from build123d import *

# Parameters (mm, degrees)
EXTRUDE_1_DEPTH           = 6
FILLET_1_R                = 3
HOLE_WIZARD_2_D           = 4.5
HOLE_WIZARD_2_CBORE_D     = 8
HOLE_WIZARD_2_CBORE_DEPTH = 4.6
CHAMFER_1_SIZE            = 1


with BuildPart() as part:
    # 草图1 → 旋转1 (revolve)
    with BuildSketch(Plane.XY):
        Polygon((-6, 10.5), (-6, 18), (0, 18), (0, 14), (4, 14), (4, 11), (-3, 11), (-3, 10.5), align=None)
    revolve(axis=Axis((-10.541189269, 0, 0), (1, 0, 0)))

    # 草图5 → 凸台-拉伸1 (add)
    with BuildSketch(Plane.ZY.offset(6)):
        with BuildLine():
            ThreePointArc((-2.6e-08, 18), (12.727922052, 12.72792207), (18, 0))
            Line((18, 0), (18, 18))
            Line((18, 18), (-2.6e-08, 18))
        make_face()
        with BuildLine():
            Line((-18, 18), (-18, 3.1e-08))
            ThreePointArc((-18, 3.1e-08), (-12.72792206, 12.727922063), (-2.6e-08, 18))
            Line((-2.6e-08, 18), (-18, 18))
        make_face()
        with BuildLine():
            Line((-18, 3.1e-08), (-18, -18))
            Line((-18, -18), (0, -18))
            ThreePointArc((0, -18), (-12.727922072, -12.727922051), (-18, 3.1e-08))
        make_face()
        with BuildLine():
            ThreePointArc((18, 0), (12.727922061, -12.727922061), (0, -18))
            Line((0, -18), (18, -18))
            Line((18, -18), (18, 0))
        make_face()
    extrude(amount=-EXTRUDE_1_DEPTH)

    # 圆角1
    fillet_1_edges = [part.edges().sort_by_distance(p)[0] for p in [
        (-3, 18, 18),
        (-3, 18, -18),
        (-3, -18, -18),
        (-3, -18, 18),
    ]]
    fillet(fillet_1_edges, radius=FILLET_1_R)

    # 打孔尺寸(%根据)内六角圆柱头螺钉的类型2 (through all)
    with Locations(Plane.ZY.offset(6)):
        with Locations((-13, 13), (13, 13), (13, -13), (-13, -13)):
            CounterBoreHole(HOLE_WIZARD_2_D / 2, HOLE_WIZARD_2_CBORE_D / 2, HOLE_WIZARD_2_CBORE_DEPTH)

    # 倒角1
    chamfer_1_edges = [part.edges().sort_by_distance(p)[0] for p in [
        (4, -11, 0),
    ]]
    chamfer(chamfer_1_edges, length=CHAMFER_1_SIZE)


solid = part.part
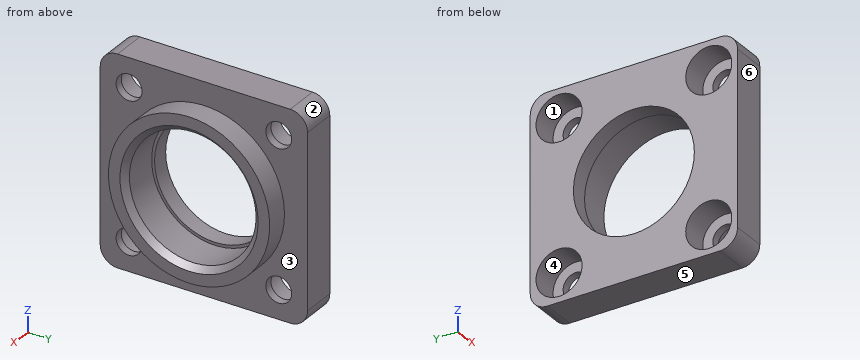
Geometry check sheet. Reference: the model listing, model coordinates, mm. Face numbers are marked on the shaded views. A direction names the side the tool comes from. Give positions to 0.01 mm unless a question says otherwise; leave off trailing zeros. Loops run counter-clockwise (first coordinate to the right, second up) from the corner with the lowest first, then second, coordinate; pieces in that order, holes last. Notation, with made-up numbers: (-29, 0.5) -> (0, 0.5) arc R19 cw to (0, 7.5) -> close; hole circle Ø7 at (0.25, -34). An arc over 180 degrees is marked (long way). Answer in a Markdown table with one row per item. Add a question column.
1) Material ranges on probe 1 along Y at (x, z) = (-3.7, 13); probe 2 along Z at (x, y) = (-1.8, 0); probe 3 along Y at (x, z) = (-0.65, -13), recorded low to high. Write a range as from..to.
2) Set-up check for the marked faces 1, 2 and 3: record each of +Z, -Z, +X, -X, +Y, -Y from which the full face is reachable in a straight line by a thin tool's end or side.
3) Draft check along Z on the marked faces 4, 5 and 6. Enter one of: pulls with the +Z half, pulls with the -Z half, needs draft (parallel to the pull), parting line crosses it, or undercut.
4) Cross-section at A-A on y = 0. Record the boundary of the cut face in (x, z).
5) Cross-section at D-D on y = -13. Record the boundary of the cut face in (x, z), and give its area (3 significant figures).
6) Gauge pin test, flat ends, axial feed: P1, Ø20, axis at y = 0, z = 0, coming from the -X side; P2, Ø7, axis at y = -13, z = -13, coming from the +X side. Record the tip position at first contact, or that the pin passes through.
7) Cross-section at B-B on x = -5. Record the boundary of the cut face in (y, z), and give its area (3 significant figures).
Outcome:
| question | item | result |
|---|---|---|
| 1 | probe 1 | y = -18..-17, -9..9, 17..18 |
| 1 | probe 2 | z = -18..-11, 11..18 |
| 1 | probe 3 | y = -18..-15.25, -10.75..10.75, 15.25..18 |
| 2 | face 1 | -X |
| 2 | face 2 | +Z, +X, -X, +Y |
| 2 | face 3 | +X |
| 3 | face 4 | undercut |
| 3 | face 5 | pulls with the -Z half |
| 3 | face 6 | needs draft |
| 4 | outline | (-6, -18) -> (0, -18) -> (0, -14) -> (4, -14) -> (4, -12) -> (3, -11) -> (-3, -11) -> (-3, -10.5) -> (-6, -10.5) -> close; (-6, 10.5) -> (-3, 10.5) -> (-3, 11) -> (3, 11) -> (4, 12) -> (4, 14) -> (0, 14) -> (0, 18) -> (-6, 18) -> close |
| 5 | outline | (-6, -18) -> (0, -18) -> (0, -15.25) -> (-1.4, -15.25) -> (-1.4, -17) -> (-6, -17) -> close; (-6, -9) -> (-1.4, -9) -> (-1.4, -10.75) -> (0, -10.75) -> (0, -5.2) -> (4, -5.2) -> (4, 5.2) -> (0, 5.2) -> (0, 10.75) -> (-1.4, 10.75) -> (-1.4, 9) -> (-6, 9) -> close; (-6, 17) -> (-1.4, 17) -> (-1.4, 15.25) -> (0, 15.25) -> (0, 18) -> (-6, 18) -> close |
| 5 | area | 171 mm^2 |
| 6 | P1 | passes through |
| 6 | P2 | stops at x = 0 |
| 7 | outline | (-18, -15) arc R3 ccw to (-15, -18) -> (15, -18) arc R3 ccw to (18, -15) -> (18, 15) arc R3 ccw to (15, 18) -> (-15, 18) arc R3 ccw to (-18, 15) -> close; hole circle Ø8 at (-13, -13); hole circle Ø8 at (-13, 13); hole circle Ø21 at (0, 0); hole circle Ø8 at (13, -13); hole circle Ø8 at (13, 13) |
| 7 | area | 741 mm^2 |
